Check sheet for the modelled part. Datum: model origin and axes. Units: mm. Face numbers are marked on the shaded views. A direction names the side the tool comes from. Round coordinates to 2 decimals unless told otherwise and drop trailing zeros. Order: outer loops, then holes, each group sorted by start corner. A loop starts at its lowest first (then second) coordinate and runs counter-clockwise, first axis right, second up. Notation, with made-up numbers: (72, -38.75) -> (86, -38.75) arc R24 ccw to (86, 0.25) -> close; hole circle Ø7 at (-6.5, 24.25). An arc over 180 degrees is marked (long way). Answer in a Markdown table with one row per item. Add a question column.
1. Depth check by flat-ended pin: P1, Ø2, axis at x = 1.5, y = 3.5, coming from the -Z side; P2, Ø2, axis at x = -2.5, y = -1.5, coming from the +Z side; P3, Ø3, axis at y = -1.5, z = 50, coming from the -X side; P4, Ø5, axis at x = -2, z = 48.5, coming from the +Y side. Enter the tip coordinate at first touch or a pass-through.
2. Sectioned sample at B-B, the plane y = 4. Record the boundary of the cut face in (x, z), then the cut area to 3 significant figures.
3. Sectioned sample at A-A, the plane x = 0. Record the boundary of the cut face in (y, z).
4. Draft check along X on the marked faces 4, 5 and 6. Enter one of: +X half, -X half, draft (parallel to the pull), parting line (faces both ways), or undercut.
5. Sectioned sample at D-D, the plane y = -2.5. Record the boundary of the cut face in (x, z), then the cut area to 3 significant figures.
6. Material ranges on L1, parallel to Y at x = 2.5, z = 4; L2, parallel to Y at x = 0, z = 34.5; L3, parallel to Z at x = -4.75, y = -7.75, recorded low to high. Write a range as from..to.
7. Sectioned sample at C-C, the plane z = 19.5. Record the boundary of the cut face in (x, y), then the cut area to 3 significant figures.
8. Access from +Z, -Z, +X, -X, +Y, -Y to the whole of each face (thin tool, end or side, straight path). Record for the marked faces 1, 2 and 3.
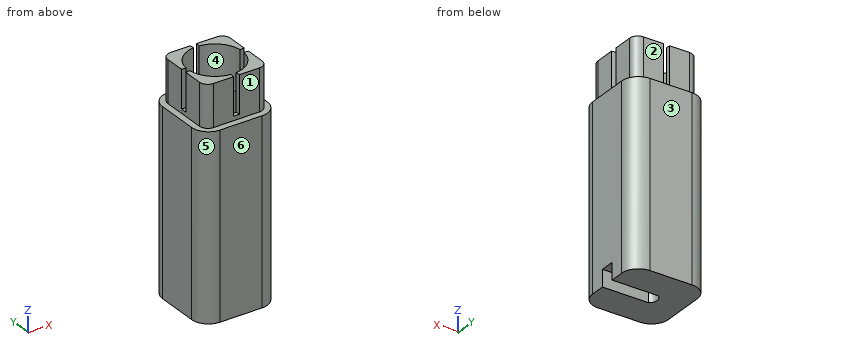
```python
from build123d import *

# Parameters (mm, degrees)
BOSS_EXTRUDE1_DEPTH = 43.61
SKETCH3_R           = 6.5
BOSS_EXTRUDE2_DEPTH = 10
CUT_EXTRUDE3_DEPTH  = 4
CUT_EXTRUDE6_DEPTH  = 2
CUT_EXTRUDE7_DEPTH  = 9
CIRPATTERN1_COUNT   = 4
SKETCH12_R          = 6.5
CUT_EXTRUDE8_DEPTH  = 37.61


with BuildPart() as part:
    # Sketch1 → Boss-Extrude1 (new body)
    with BuildSketch(Plane.XY):
        with BuildLine():
            Line((-5.05, 9.05), (5.05, 9.05))
            ThreePointArc((5.05, 9.05), (7.878427125, 7.878427125), (9.05, 5.05))
            Line((9.05, 5.05), (9.05, -5.05))
            ThreePointArc((9.05, -5.05), (7.878427125, -7.878427125), (5.05, -9.05))
            Line((5.05, -9.05), (-5.05, -9.05))
            ThreePointArc((-5.05, -9.05), (-7.878427125, -7.878427125), (-9.05, -5.05))
            Line((-9.05, -5.05), (-9.05, 5.05))
            ThreePointArc((-9.05, 5.05), (-7.878427125, 7.878427125), (-5.05, 9.05))
        make_face()
    extrude(amount=BOSS_EXTRUDE1_DEPTH)

    # Sketch3 → Boss-Extrude2 (add)
    with BuildSketch(Plane.XY.offset(43.61)):
        with BuildLine():
            Line((-5.509134554, -7.499739888), (5.490865446, -7.499739888))
            ThreePointArc((5.490865446, -7.499739888), (6.905079008, -6.91395345), (7.490865446, -5.499739888))
            Line((7.490865446, -5.499739888), (7.490865446, 5.500260112))
            ThreePointArc((7.490865446, 5.500260112), (6.905079008, 6.914473675), (5.490865446, 7.500260112))
            Line((5.490865446, 7.500260112), (-5.509134554, 7.500260112))
            ThreePointArc((-5.509134554, 7.500260112), (-6.923348116, 6.914473675), (-7.509134554, 5.500260112))
            Line((-7.509134554, 5.500260112), (-7.509134554, -5.499739888))
            ThreePointArc((-7.509134554, -5.499739888), (-6.923348116, -6.91395345), (-5.509134554, -7.499739888))
        make_face()
        with Locations((-0.009134554, 0.000260112)):
            Circle(SKETCH3_R, mode=Mode.SUBTRACT)
    extrude(amount=BOSS_EXTRUDE2_DEPTH)

    # Sketch6 → Cut-Extrude3 (cut)
    with BuildSketch(Plane.XY):
        with BuildLine():
            Line((-2, -1.68), (2, -1.68))
            Line((2, -1.68), (9.05, -1.68))
            Line((9.05, -1.68), (9.05, 1.68))
            Line((9.05, 1.68), (2, 1.68))
            Line((2, 1.68), (-2, 1.68))
            ThreePointArc((-2, 1.68), (-2.914827203, 0), (-2, -1.68))
        make_face()
    extrude(amount=CUT_EXTRUDE3_DEPTH, mode=Mode.SUBTRACT)

    # Sketch10 → Cut-Extrude6 (cut)
    with BuildSketch(Plane(origin=(0, 0, 4), x_dir=(-1, 0, 0), z_dir=(0, 0, -1))):
        with BuildLine():
            Line((-2.7, 1.68), (2, 1.68))
            ThreePointArc((2, 1.68), (2.914827203, 0), (2, -1.68))
            Line((2, -1.68), (-2.7, -1.68))
            Line((-2.7, -1.68), (-2.7, 1.68))
        make_face()
    extrude(amount=-CUT_EXTRUDE6_DEPTH, mode=Mode.SUBTRACT)

    # Sketch11 → Cut-Extrude7 (cut)
    with BuildSketch(Plane.XY.offset(53.61)):
        Polygon((0, 0), (7.490865446, 0.75), (7.490865446, -0.75), align=None)
    cut_extrude7 = extrude(amount=-CUT_EXTRUDE7_DEPTH, mode=Mode.SUBTRACT)

    # CirPattern1: Cut-Extrude7 ×4 about axis
    cirpattern1_axis = Axis((-0.009134554, 0.000260112, 0), (0, 0, 1))
    for i in range(1, CIRPATTERN1_COUNT):
        add(cut_extrude7.rotate(cirpattern1_axis, i * 360 / CIRPATTERN1_COUNT), mode=Mode.SUBTRACT)

    # Sketch12 → Cut-Extrude8 (cut)
    with BuildSketch(Plane.XY.offset(43.61)):
        with Locations((0, 0.192488852)):
            Circle(SKETCH12_R)
    extrude(amount=-CUT_EXTRUDE8_DEPTH, mode=Mode.SUBTRACT)


solid = part.part
```
Answer key:
| question | item | result |
|---|---|---|
| 1 | P1 | stops at z = 0 |
| 1 | P2 | stops at z = 6 |
| 1 | P3 | stops at x = -7.51 |
| 1 | P4 | stops at y = 7.5 |
| 2 | outline | (-9.05, 0) -> (9.05, 0) -> (9.05, 43.61) -> (7.49, 43.61) -> (7.49, 53.61) -> (5.11, 53.61) -> (5.11, 43.61) -> (5.27, 43.61) -> (5.27, 6) -> (-5.27, 6) -> (-5.27, 43.61) -> (-5.13, 43.61) -> (-5.13, 53.61) -> (-7.51, 53.61) -> (-7.51, 43.61) -> (-9.05, 43.61) -> close |
| 2 | area | 441 mm² |
| 3 | outline | (-9.05, 0) -> (-1.68, 0) -> (-1.68, 6) -> (-6.31, 6) -> (-6.31, 43.61) -> (-6.5, 43.61) -> (-6.5, 44.61) -> (-7.5, 44.61) -> (-7.5, 43.61) -> (-9.05, 43.61) -> close; (1.68, 0) -> (9.05, 0) -> (9.05, 43.61) -> (7.5, 43.61) -> (7.5, 44.61) -> (6.5, 44.61) -> (6.5, 43.61) -> (6.69, 43.61) -> (6.69, 6) -> (1.68, 6) -> close |
| 4 | face 4 | undercut |
| 4 | face 5 | -X half |
| 4 | face 6 | draft |
| 5 | outline | (-9.05, 0) -> (9.05, 0) -> (9.05, 43.61) -> (7.49, 43.61) -> (7.49, 53.61) -> (5.99, 53.61) -> (5.99, 43.61) -> (5.92, 43.61) -> (5.92, 6) -> (-5.92, 6) -> (-5.92, 43.61) -> (-6.01, 43.61) -> (-6.01, 53.61) -> (-7.51, 53.61) -> (-7.51, 43.61) -> (-9.05, 43.61) -> close |
| 5 | area | 374 mm² |
| 6 | L1 | y = -9.05..-1.68, 1.68..9.05 |
| 6 | L2 | y = -9.05..-6.31, 6.69..9.05 |
| 6 | L3 | z = 0..43.61 |
| 7 | outline | (-9.05, -5.05) arc R4 ccw to (-5.05, -9.05) -> (5.05, -9.05) arc R4 ccw to (9.05, -5.05) -> (9.05, 5.05) arc R4 ccw to (5.05, 9.05) -> (-5.05, 9.05) arc R4 ccw to (-9.05, 5.05) -> close; hole circle Ø13 at (0, 0.19) |
| 7 | area | 181 mm² |
| 8 | face 1 | +Z, +X, -X, -Y |
| 8 | face 2 | +Z, +X, -X, +Y |
| 8 | face 3 | +Z, -Z, +X, -X, +Y |
